Work out the finished part from the listing and answer in its coordinate system (mm). Face numbers are marked on the shaded views. A direction names the side the tool comes from. Give positions to 0.01 mm unless a question says otherwise; leave off trailing zeros. Loops run counter-clockwise (first coordinate to the right, second up) from the corner with the lowest first, then second, coordinate; pieces in that order, holes last. Notation, with made-up numbers: (20, 4) - (68, 4) arc R13 cw to (68, 26) - close; hole circle Ø5 at (82.5, -13). An arc over 180 degrees is marked (long way). One line per question, with ' | ' between items.
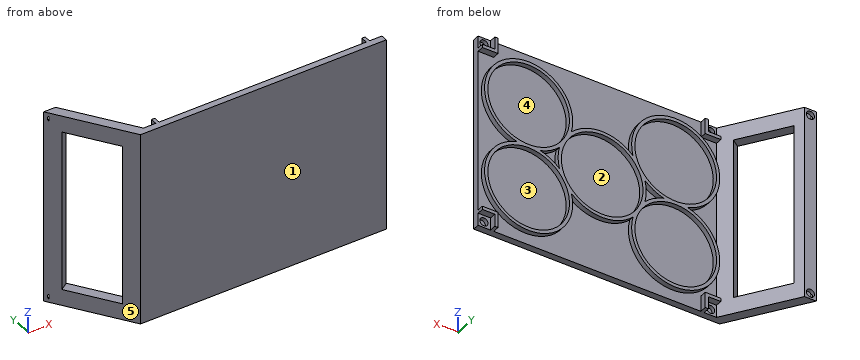
from build123d import *

# Parameters (mm, degrees)
SKETCH1_W           = 73.033321
SKETCH1_H           = 59.5
BOSS_EXTRUDE1_DEPTH = 2
SKETCH2_R           = 13.5
SKETCH2_R_2         = 12.5
BOSS_EXTRUDE2_DEPTH = 1.5
SKETCH3_R           = 1.25
CUT_EXTRUDE1_DEPTH  = 1.2
BOSS_EXTRUDE3_DEPTH = 59.5
SKETCH5_R           = 1.25
CUT_EXTRUDE2_DEPTH  = 1.2
SKETCH7_W           = 49.5
SKETCH7_H           = 16.666550208
CUT_EXTRUDE4_DEPTH  = 3.6
BOSS_EXTRUDE4_DEPTH = 2


with BuildPart() as part:
    # Sketch1 → Boss-Extrude1 (new body)
    with BuildSketch(Plane(origin=(0, 0, 0), x_dir=(1, 0, 0), z_dir=(0, 1, 0))):
        with Locations((-151.204244356, -15.021595707)):
            Rectangle(SKETCH1_W, SKETCH1_H)
    extrude(amount=BOSS_EXTRUDE1_DEPTH)

    # Sketch2 → Boss-Extrude2 (add)
    # profile 1 of 5: a face of its own
    with BuildSketch(Plane(origin=(0, 2, 0), x_dir=(1, 0, 0), z_dir=(0, 1, 0))):
        with Locations((-129.187583856, -28.021595707)):
            Circle(SKETCH2_R)
        with Locations(Location((-129.187583856, -28.021595707, 0), (0, 0, 270))):
            Circle(SKETCH2_R_2, mode=Mode.SUBTRACT)
    # profile 2 of 5: a face of its own
    with BuildSketch(Plane(origin=(0, 2, 0), x_dir=(1, 0, 0), z_dir=(0, 1, 0))):
        with Locations((-129.187583856, -2.021595707)):
            Circle(SKETCH2_R)
        with Locations(Location((-129.187583856, -2.021595707, 0), (0, 0, 270))):
            Circle(SKETCH2_R_2, mode=Mode.SUBTRACT)
    # profile 3 of 5: a face of its own
    with BuildSketch(Plane(origin=(0, 2, 0), x_dir=(1, 0, 0), z_dir=(0, 1, 0))):
        with Locations((-151.704244355, -15.021595707)):
            Circle(SKETCH2_R)
        with Locations(Location((-151.704244355, -15.021595707, 0), (0, 0, 270))):
            Circle(SKETCH2_R_2, mode=Mode.SUBTRACT)
    # profile 4 of 5: a face of its own
    with BuildSketch(Plane(origin=(0, 2, 0), x_dir=(1, 0, 0), z_dir=(0, 1, 0))):
        with Locations((-174.220904853, -2.021595707)):
            Circle(SKETCH2_R)
        with Locations(Location((-174.220904853, -2.021595707, 0), (0, 0, 270))):
            Circle(SKETCH2_R_2, mode=Mode.SUBTRACT)
    # profile 5 of 5: a face of its own
    with BuildSketch(Plane(origin=(0, 2, 0), x_dir=(1, 0, 0), z_dir=(0, 1, 0))):
        with Locations((-174.220904853, -28.021595707)):
            Circle(SKETCH2_R)
        with Locations(Location((-174.220904853, -28.021595707, 0), (0, 0, 270))):
            Circle(SKETCH2_R_2, mode=Mode.SUBTRACT)
    extrude(amount=BOSS_EXTRUDE2_DEPTH)

    # Sketch3 → Cut-Extrude1 (cut)
    with BuildSketch(Plane(origin=(0, 2, 0), x_dir=(1, 0, 0), z_dir=(0, 1, 0))):
        with Locations(Location((-185.920904856, 12.928404293, 0), (0, 0, 270))):
            Circle(SKETCH3_R)
        with Locations(Location((-185.920904856, -42.971595707, 0), (0, 0, 270))):
            Circle(SKETCH3_R)
        with Locations(Location((-116.487583856, -42.971595707, 0), (0, 0, 270))):
            Circle(SKETCH3_R)
        with Locations(Location((-116.487583856, 12.928404293, 0), (0, 0, 270))):
            Circle(SKETCH3_R)
    extrude(amount=-CUT_EXTRUDE1_DEPTH, mode=Mode.SUBTRACT)

    # Sketch4 → Boss-Extrude3 (add)
    with BuildSketch(Plane.XY.offset(44.771595707)):
        Polygon((-201.420904856, 22), (-187.720904856, 2), (-187.720904856, 0), (-189.950904856, 0), (-191.320904856, 2), (-205.020904856, 22), align=None)
    extrude(amount=-BOSS_EXTRUDE3_DEPTH)

    # Sketch5 → Cut-Extrude2 (cut)
    with BuildSketch(Plane(origin=(0, 22, 0), x_dir=(1, 0, 0), z_dir=(0, 1, 0))):
        with Locations(Location((-203.220904856, 12.928404293, 0), (0, 0, 180))):
            Circle(SKETCH5_R)
        with Locations(Location((-203.220904856, -42.971595707, 0), (0, 0, 180))):
            Circle(SKETCH5_R)
    extrude(amount=-CUT_EXTRUDE2_DEPTH, mode=Mode.SUBTRACT)

    # Sketch7 → Cut-Extrude4 (cut)
    with BuildSketch(Plane(origin=(-129.286463854, -88.56122774, 0), x_dir=(0, 0, 1), z_dir=(-0.8250036029532889, -0.5651274680230048, 0))):
        with Locations((15.021595707, 120.679749014)):
            Rectangle(SKETCH7_W, SKETCH7_H)
    extrude(amount=-CUT_EXTRUDE4_DEPTH, mode=Mode.SUBTRACT)

    # Sketch8 → Boss-Extrude4 (add)
    with BuildSketch(Plane(origin=(0, 2, 0), x_dir=(1, 0, 0), z_dir=(0, 1, 0))):
        Polygon((-182.920904856, 9.928404293), (-182.920904856, 14.728404293), (-183.920904856, 14.728404293), (-183.920904856, 10.928404293), (-187.720904856, 10.928404293), (-187.720904856, 9.928404293), align=None)
        Polygon((-183.920904856, -40.971595707), (-183.920904856, -44.771595707), (-182.920904856, -44.771595707), (-182.920904856, -39.971595707), (-187.720904856, -39.971595707), (-187.720904856, -40.971595707), align=None)
        Polygon((-119.487583856, -39.971595707), (-119.487583856, -44.771595707), (-118.487583856, -44.771595707), (-118.487583856, -40.971595707), (-114.687583856, -40.971595707), (-114.687583856, -39.971595707), align=None)
        Polygon((-119.487583856, 9.928404293), (-114.687583856, 9.928404293), (-114.687583856, 10.928404293), (-118.487583856, 10.928404293), (-118.487583856, 14.728404293), (-119.487583856, 14.728404293), align=None)
    extrude(amount=BOSS_EXTRUDE4_DEPTH)


solid = part.part
1. Find section D-D on x = -137. Write down the section's boundary in (y, z), then the cut area to 3 significant figures.
Evaluation:
outline: (0, -14.73) - (2, -14.73) - (2, -8.99) - (3.5, -8.99) - (3.5, -7.74) - (2, -7.74) - (2, 11.78) - (3.5, 11.78) - (3.5, 13.03) - (2, 13.03) - (2, 17.01) - (3.5, 17.01) - (3.5, 18.26) - (2, 18.26) - (2, 37.78) - (3.5, 37.78) - (3.5, 39.03) - (2, 39.03) - (2, 44.77) - (0, 44.77) - close | area: 127 mm2
2. Find section A-A on z = 34.5. Write down the section's boundary in (x, y) (3 decimals).
Evaluation:
outline: (-205.021, 22) - (-202.195, 17.875) - (-199.745, 19.553) - (-201.421, 22) - close; (-192.777, 4.125) - (-189.951, 0) - (-114.688, 0) - (-114.688, 2) - (-117.344, 2) - (-117.344, 3.5) - (-118.497, 3.5) - (-118.497, 2) - (-139.878, 2) - (-139.878, 3.5) - (-141.032, 3.5) - (-141.032, 2) - (-162.377, 2) - (-162.377, 3.5) - (-163.531, 3.5) - (-163.531, 2) - (-184.911, 2) - (-184.911, 3.5) - (-186.065, 3.5) - (-186.065, 2) - (-187.721, 2) - (-190.326, 5.803) - close
3. Which of the six approach directions +Z, -Z, +X, -X, +Y, -Y give full straight-line access (tool end or side, diameter ignored) to the marked faces 4 and 5?
Evaluation:
face 4: +Y | face 5: +Z, -Z, -X, -Y
4. Find section B-B on y = 14.75. Write down the section's boundary in (x, z).
Evaluation:
outline: (-200.05, -14.73) - (-196.45, -14.73) - (-196.45, -9.73) - (-200.05, -9.73) - close; (-200.05, 39.77) - (-196.45, 39.77) - (-196.45, 44.77) - (-200.05, 44.77) - close
5. Consider L1, parallel to Y at x = -151, z = 5; L2, parallel to Z at x = -120, y = 3.25; L3, parallel to Y at x = -167.5, z = 16.5. Determine where each line is inside the solid, lowest interval first.
Evaluation:
L1: 0 to 2 | L2: -7.87 to -6.45, 10.5 to 11.91, 18.13 to 19.55, 36.5 to 37.91 | L3: 0 to 3.5
6. Flat-ended cylindrical pins translate along their axes: pin 1 (1.1 mm diameter, centred on x = -116.5, z = -13.5, fed in from +Y); pin 2 (0.6 mm diameter, centred on x = -116.5, y = 2.5, fed in from -Z); pin 3 (0.6 mm diameter, centred on x = -117.5, y = 3.5, fed in from +Z); pin 4 (2 mm diameter, centred on x = -155, y = 6, fed in from +Z). Find the tip coordinate at first contact, or state that the pin passes through.
Evaluation:
pin 1: y = 0.8 | pin 2: z = -10.93 | pin 3: z = 40.97 | pin 4: through
7. Find section C-C on x = -175.5. Write down the section's boundary in (y, z).
Evaluation:
outline: (0, -14.73) - (2, -14.73) - (2, -11.42) - (3.5, -11.42) - (3.5, -10.41) - (2, -10.41) - (2, 14.46) - (3.5, 14.46) - (3.5, 15.59) - (2, 15.59) - (2, 40.46) - (3.5, 40.46) - (3.5, 41.46) - (2, 41.46) - (2, 44.77) - (0, 44.77) - close
8. Determine the mould class of the marked faces 1, 2 and 3 for opening direction Z: +Z half, -Z half, draft (parallel to the pull), parting line (faces both ways), or undercut.
Evaluation:
face 1: draft | face 2: undercut | face 3: undercut
